Work out the finished part from the listing and answer in its coordinate system (mm). Round coordinates to 2 decimals unless told otherwise and drop trailing zeros. Order: outer loops, then holes, each group sorted by start corner. A loop starts at its lowest first (then second) coordinate and runs counter-clockwise, first axis right, second up. Notation, with made-up numbers: M -27,23.25 L -20,23.25 A12 cw -20,40.25 Z; hole C 54,9.25 d9. An arc over 180 degrees is marked long. Return JSON: item names as keys, results as strings.
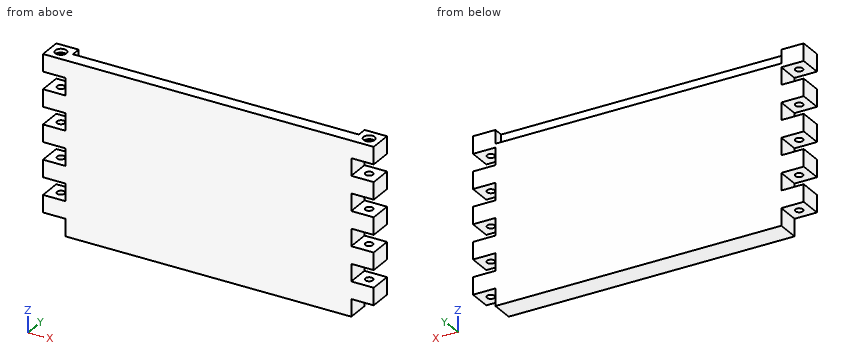
from build123d import *

# Parameters (mm, degrees)
F1_DEPTH       = 30
F3_D           = 10
F3_CBORE_D     = 15
F3_CBORE_DEPTH = 5
F2_W           = 382
F2_H           = 13
F4_DEPTH       = 18


with BuildPart() as f1:
    # F0 (on Front) → F1 (new body)
    with BuildSketch(Plane.XZ):
        Polygon((221, 92), (221, 115), (-221, 115), (-221, 92), (-191, 92), (-191, 69), (-221, 69), (-221, 46), (-191, 46), (-191, 23), (-221, 23), (-221, 0), (-191, 0), (-191, -23), (-221, -23), (-221, -46), (-191, -46), (-191, -69), (-221, -69), (-221, -92), (-191, -92), (-191, -115), (191, -115), (191, -92), (221, -92), (221, -69), (191, -69), (191, -46), (221, -46), (221, -23), (191, -23), (191, 0), (221, 0), (221, 23), (191, 23), (191, 46), (221, 46), (221, 69), (191, 69), (191, 92), align=None)
    extrude(amount=F1_DEPTH)

    # F3 (through all)
    with Locations(Plane.XY.offset(115)):
        with Locations((-206, -15), (206, -15)):
            CounterBoreHole(F3_D / 2, F3_CBORE_D / 2, F3_CBORE_DEPTH)

    # F2 (on face) → F4 (cut)
    with BuildSketch(Plane.XY.offset(115)):
        with Locations((0, -6.5)):
            Rectangle(F2_W, F2_H)
    extrude(amount=-F4_DEPTH, mode=Mode.SUBTRACT)


solid = f1.part
Item 1: Find section A-A (x = -206). State how many separate pieces and enclosed holes the cut face has, plus the area to 4 significant figures.
Output:
{"separate pieces": "10", "enclosed holes": "0", "area": "2,275 mm^2"}
Item 2: Find section B-B (x = 11.5). Determine the outline of the cut face in (y, z).
Output:
{"outline": "M -30,-115 L 0,-115 L 0,97 L -13,97 L -13,115 L -30,115 Z"}
Item 3: Consider line 1 along Z through (x, y) = (198.5, -6.5); line 2 along Y through (x, z) = (206, 103); line 3 along X through (y, z) = (-10.75, -9). Determine where each line is inside the solid, lowest interval first. Write a range as [from, to].
Output:
{"line 1": "z = [-92, -69], [-46, -23], [0, 23], [46, 69], [92, 115]", "line 2": "y = [-30, -20], [-10, 0]", "line 3": "x = [-191, 191]"}
Item 4: Each of these flat-tipped pins is pushed along its axis until it touches: pin 1 (11.5 mm diameter, centred on x = -206, y = -15, fed in from +Z); pin 2 (7 mm diameter, centred on y = -17.5, z = -9, fed in from +X); pin 3 (6 mm diameter, centred on x = 206, y = -15, fed in from -Z); pin 4 (3 mm diameter, centred on x = -44.5, y = -8, fed in from +Z). Where does it stop, or does it pass through?
Output:
{"pin 1": "stops at z = 110", "pin 2": "stops at x = 191", "pin 3": "passes through", "pin 4": "stops at z = 97"}
